The model under review builds one solid part; all positions refer to its coordinate system, in mm. Give positions to 0.01 mm unless a question says otherwise; leave off trailing zeros. Write each loop counter-clockwise with the first axis right and the second up, starting at its lowest first coordinate (ties: lowest second). Pieces come first, ordered by that corner, then holes.
from build123d import *

# Parameters (mm, degrees)
SKETCH1_W           = 57.404
SKETCH1_H           = 57.404
SKETCH1_R           = 1.524
BOSS_EXTRUDE1_DEPTH = 5.08
SKETCH2_R           = 2.667
CUT_EXTRUDE1_DEPTH  = 2.54
SKETCH3_R           = 1.524
CUT_EXTRUDE2_DEPTH  = 41.90740774


with BuildPart() as part:
    # Sketch1 → Boss-Extrude1 (new body)
    with BuildSketch(Plane.XY):
        Rectangle(SKETCH1_W, SKETCH1_H)
        with Locations(Location((-24.13, 24.13, 0), (0, 0, 180))):
            Circle(SKETCH1_R, mode=Mode.SUBTRACT)
        with Locations(Location((-24.13, -24.13, 0), (0, 0, 180))):
            Circle(SKETCH1_R, mode=Mode.SUBTRACT)
        with Locations(Location((24.13, -24.13, 0), (0, 0, 180))):
            Circle(SKETCH1_R, mode=Mode.SUBTRACT)
        with Locations(Location((24.13, 24.13, 0), (0, 0, 180))):
            Circle(SKETCH1_R, mode=Mode.SUBTRACT)
    extrude(amount=BOSS_EXTRUDE1_DEPTH)

    # Sketch2 → Cut-Extrude1 (cut)
    with BuildSketch(Plane.XY.offset(5.08)):
        with Locations((-24.13, -24.13)):
            Circle(SKETCH2_R)
        with Locations((-24.13, 24.13)):
            Circle(SKETCH2_R)
        with Locations((24.13, 24.13)):
            Circle(SKETCH2_R)
        with Locations((24.13, -24.13)):
            Circle(SKETCH2_R)
    extrude(amount=-CUT_EXTRUDE1_DEPTH, mode=Mode.SUBTRACT)

    # Sketch3 → Cut-Extrude2 (cut, through all)
    with BuildSketch(Plane.XY.offset(5.08)):
        with Locations((0, 6.35)):
            Circle(SKETCH3_R)
    extrude(amount=-CUT_EXTRUDE2_DEPTH, mode=Mode.SUBTRACT)


solid = part.part
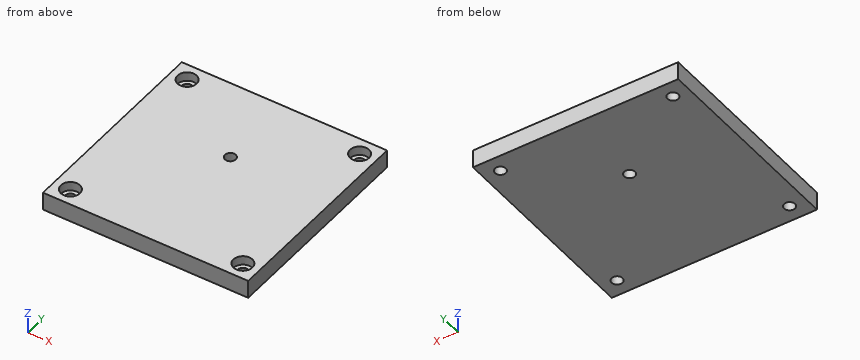
1) Consider section A-A, the plane x = -24.13. Give the boundary of the cut face in (y, z).
2) Consider section B-B, the plane y = 6.35. Give the boundary of the cut face in (x, z), then the cut area to 3 significant figures.
3) To check wall thickness, follow probe 1 along Y at (x, z) = (24.13, 4.35); probe 2 along X at (y, z) = (-24.13, 1.1). State the ranges of each line that lie inside material, in increasing order.
4) Insertion check: pin 1 (3.5 mm diameter, centred on x = 24.13, y = 24.13, fed in from +Z). The pin has a flat end and moves straight along its axis. Give the tip position at first contact, or say it passes through.
5) Consider section C-C, the plane z = 3.85. Give the boundary of the cut face in (x, y), then the cut area to 3 significant figures.
Answer block:
1. outline: (-28.7, 0) - (-25.65, 0) - (-25.65, 2.54) - (-26.8, 2.54) - (-26.8, 5.08) - (-28.7, 5.08) - close; (-22.61, 0) - (22.61, 0) - (22.61, 2.54) - (21.46, 2.54) - (21.46, 5.08) - (-21.46, 5.08) - (-21.46, 2.54) - (-22.61, 2.54) - close; (25.65, 0) - (28.7, 0) - (28.7, 5.08) - (26.8, 5.08) - (26.8, 2.54) - (25.65, 2.54) - close
2. outline: (-28.7, 0) - (-1.52, 0) - (-1.52, 5.08) - (-28.7, 5.08) - close; (1.52, 0) - (28.7, 0) - (28.7, 5.08) - (1.52, 5.08) - close
2. area: 276 mm2
3. probe 1: y = -28.7 to -26.8, -21.46 to 21.46, 26.8 to 28.7
3. probe 2: x = -28.7 to -25.65, -22.61 to 22.61, 25.65 to 28.7
4. pin 1: stops at z = 2.54
5. outline: (-28.7, -28.7) - (28.7, -28.7) - (28.7, 28.7) - (-28.7, 28.7) - close; hole circle Ø5.33 at (-24.13, -24.13); hole circle Ø5.33 at (-24.13, 24.13); hole circle Ø3.05 at (0, 6.35); hole circle Ø5.33 at (24.13, -24.13); hole circle Ø5.33 at (24.13, 24.13)
5. area: 3,200 mm2
